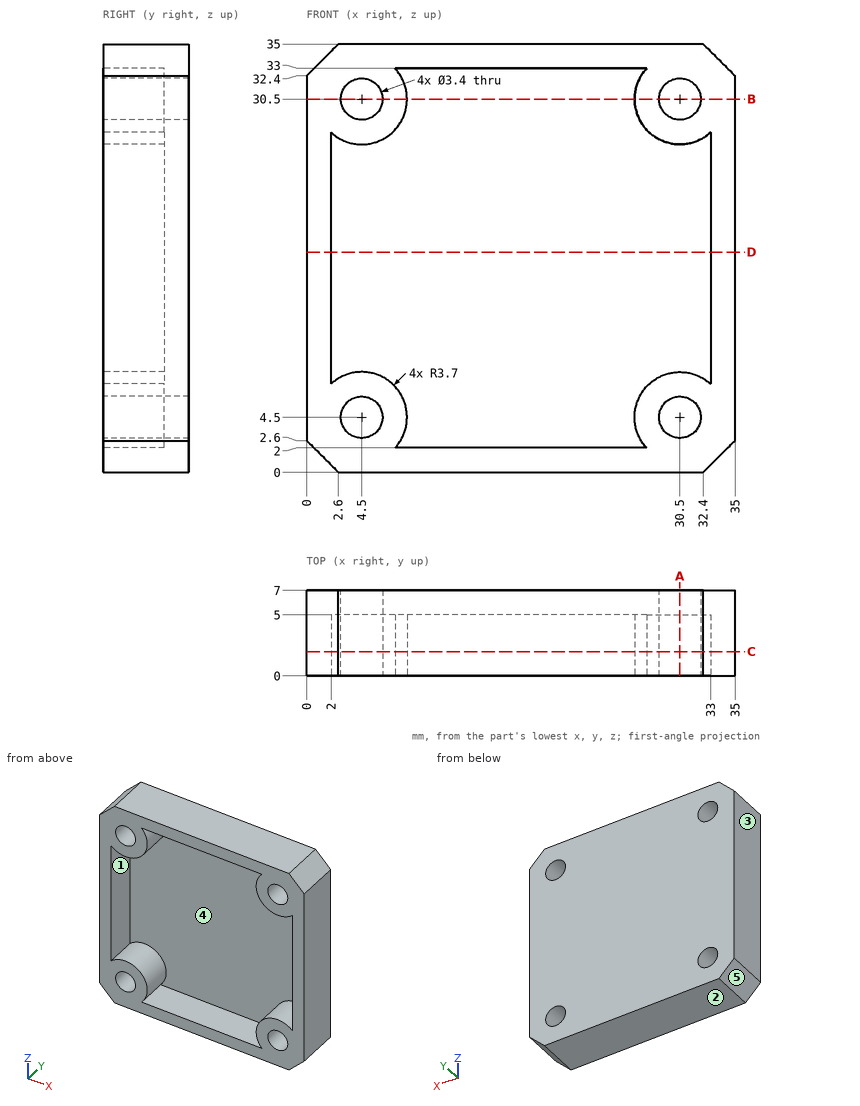
Check sheet for the drawn part. Datum: minimum x, y, z corner. Units: mm. A direction names the side the tool comes from. Coordinates: 2 decimals unless noted, no trailing zeros. Order: outer loops, then holes, each group sorted by start corner. A loop starts at its lowest first (then second) coordinate and runs counter-clockwise, first axis right, second up. Notation, with made-up numbers: (64, 63) - (101, 63) arc R36 ccw to (101, 98) - close; hole circle Ø7 at (19.25, 85.5). An arc over 180 degrees is marked (long way). Return JSON: item names as keys, results as strings.
(1) Mould release check, pull along Z, two halves, no side actions. Record for the marked faces 1, 2 and 3: pulls with the +Z half, pulls with the -Z half, needs draft (parallel to the pull), parting line crosses it, or undercut.
Filled sheet:
{"face 1": "undercut", "face 2": "pulls with the -Z half", "face 3": "needs draft"}
(2) Thickness scan on line 1 along Z through (x, y) = (4.5, 5.75); line 2 along Z through (x, y) = (30.5, 1.75); line 3 along X through (y, z) = (1.75, 11). Record the ranges inside material, lowest first.
Filled sheet:
{"line 1": "z = 0 to 2.8, 6.2 to 28.8, 32.2 to 35", "line 2": "z = 0 to 2.8, 6.2 to 8.2, 26.8 to 28.8, 32.2 to 35", "line 3": "x = 0 to 2, 33 to 35"}
(3) Go/stop test with flat-tipped pins: pin 1 (3 mm diameter, centred on x = 30.5, z = 30.5, fed in from +Y); pin 2 (5.5 mm diameter, centred on x = 4.5, z = 4.5, fed in from -Y); pin 3 (9.5 mm diameter, centred on x = 14.5, z = 19.5, fed in from -Y). Record where each tip stops, or that it passes through.
Filled sheet:
{"pin 1": "passes through", "pin 2": "stops at y = 0", "pin 3": "stops at y = 5"}
(4) Section check B-B, the plane z = 30.5. Record the cut outline in (x, y).
Filled sheet:
{"outline": "(0, 0) - (2.8, 0) - (2.8, 7) - (0, 7) - close; (6.2, 0) - (8.2, 0) - (8.2, 5) - (26.8, 5) - (26.8, 0) - (28.8, 0) - (28.8, 7) - (6.2, 7) - close; (32.2, 0) - (35, 0) - (35, 7) - (32.2, 7) - close"}
(5) Section check D-D, the plane z = 18. Record the cut outline in (x, y).
Filled sheet:
{"outline": "(0, 0) - (2, 0) - (2, 5) - (33, 5) - (33, 0) - (35, 0) - (35, 7) - (0, 7) - close"}
(6) Section check C-C, the plane y = 2. Record the cut outline in (x, z).
Filled sheet:
{"outline": "(0, 2.6) - (2.6, 0) - (32.4, 0) - (35, 2.6) - (35, 32.4) - (32.4, 35) - (2.6, 35) - (0, 32.4) - close; hole (2, 7.23) arc R3.7 cw to (7.23, 2) - (27.77, 2) arc R3.7 cw to (33, 7.23) - (33, 27.77) arc R3.7 cw to (27.77, 33) - (7.23, 33) arc R3.7 cw to (2, 27.77) - close; hole circle Ø3.4 at (4.5, 4.5); hole circle Ø3.4 at (4.5, 30.5); hole circle Ø3.4 at (30.5, 4.5); hole circle Ø3.4 at (30.5, 30.5)"}
(7) Section check A-A, the plane x = 30.5. Record the cut outline in (y, z), and give its area (3 significant figures).
Filled sheet:
{"outline": "(0, 0) - (7, 0) - (7, 2.8) - (0, 2.8) - close; (0, 6.2) - (7, 6.2) - (7, 28.8) - (0, 28.8) - (0, 26.8) - (5, 26.8) - (5, 8.2) - (0, 8.2) - close; (0, 32.2) - (7, 32.2) - (7, 35) - (0, 35) - close", "area": "104 mm^2"}
(8) Access from +Z, -Z, +X, -X, +Y, -Y to the whole of each face (thin tool, end or side, straight path). Record for the marked faces 4 and 5.
Filled sheet:
{"face 4": "-Y", "face 5": "-Z, -X, +Y, -Y"}
